For this review, use the dimensioned drawing (mm, ordinates from the lowest corner) and the shaded views. A direction names the side the tool comes from. Coordinates: 2 decimals unless noted, no trailing zeros. Loops run counter-clockwise (first coordinate to the right, second up) from the corner with the lowest first, then second, coordinate; pieces in that order, holes last. Notation, with made-up numbers: M 56.5,22 L 90.5,22 A14 cw 90.5,39 Z; hole C 6.5,-9 d1. An arc over 180 degrees is marked long. One line per item, written item: value.
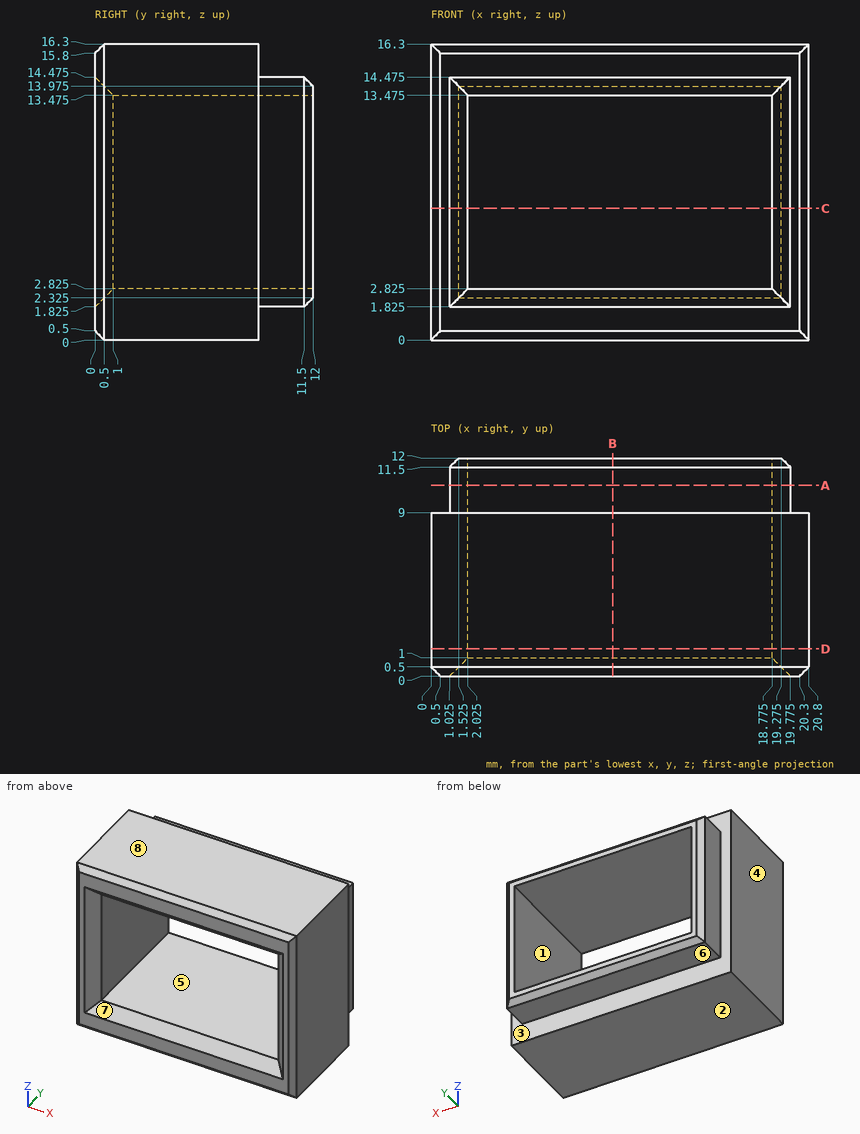
(1) Add section B-B on x = 10. State the section outline as (y, z) points (3 decimals), then the cut area to 4 significant figures.
Checks:
outline: M 0,0.5 L 0.5,0 L 9,0 L 9,1.825 L 11.5,1.825 L 12,2.325 L 12,2.825 L 1,2.825 L 0,1.825 Z; M 0,14.475 L 1,13.475 L 12,13.475 L 12,13.975 L 11.5,14.475 L 9,14.475 L 9,16.3 L 0.5,16.3 L 0,15.8 Z
area: 55.35 mm^2
(2) Add section A-A on y = 10.5. State the section outline as (x, z) points (3 decimals).
Checks:
outline: M 1.025,1.825 L 19.775,1.825 L 19.775,14.475 L 1.025,14.475 Z; hole M 2.025,2.825 L 18.775,2.825 L 18.775,13.475 L 2.025,13.475 Z
(3) Add section D-D on y = 1.5. State the section outline as (x, z) points (3 decimals).
Checks:
outline: M 0,0 L 20.8,0 L 20.8,16.3 L 0,16.3 Z; hole M 2.025,2.825 L 18.775,2.825 L 18.775,13.475 L 2.025,13.475 Z
(4) Tool access review of the marked faces 4, 5, 6, 7 and 8: name each direction out of +Z, -Z, +X, -X, +Y, -Y from which nothing blocks a thin tool from reaching the whole face with its end or side.
Checks:
face 4: +Z, -Z, -X, +Y, -Y
face 5: +Y, -Y
face 6: -Z, +X, -X, +Y
face 7: -Y
face 8: +Z, +X, -X, +Y, -Y
(5) Add section C-C on z = 7.25. State the section outline as (x, y) points (3 decimals).
Checks:
outline: M 0,0.5 L 0.5,0 L 1.025,0 L 2.025,1 L 2.025,12 L 1.525,12 L 1.025,11.5 L 1.025,9 L 0,9 Z; M 18.775,1 L 19.775,0 L 20.3,0 L 20.8,0.5 L 20.8,9 L 19.775,9 L 19.775,11.5 L 19.275,12 L 18.775,12 Z
(6) Draft analysis for pull direction Z (two halves, no side actions). For the marked faces 1, 2 and 3, state which applies: pulls with the +Z half, pulls with the -Z half, needs draft (parallel to the pull), parting line crosses it, or undercut.
Checks:
face 1: undercut
face 2: pulls with the -Z half
face 3: needs draft
(7) To check wall thickness, follow L1, parallel to X at y = 6.5, z = 5 (3 decimals); L2, parallel to Z at x = 15.5, y = 8 (3 decimals); L3, parallel to Y at x = 12.5, z = 15.25. State the ranges of each line that lie inside material, in increasing order. Write a range as [from, to].
Checks:
L1: [0, 2.025], [18.775, 20.8]
L2: [0, 2.825], [13.475, 16.3]
L3: [0, 9]
(8) Insertion check: pin 1 Ø1.2 at (y, z) = (10, 10) entering from -X (3 decimals); pin 2 Ø3 at (y, z) = (7, 8) entering from -X; pin 3 Ø2 at (x, y) = (7.5, 10.5) entering from -Z (3 decimals); pin 4 Ø2 at (y, z) = (10.5, 6) entering from +X (3 decimals). Each pin has a flat end and moves straight along its axis. Give the tip position at first contact, or say it passes through.
Checks:
pin 1: x = 1.025
pin 2: x = 0
pin 3: z = 1.825
pin 4: x = 19.775
